Build history of the part. All positions in model axes, mm. A direction names the side the tool comes from. Round coordinates to 2 decimals unless told otherwise and drop trailing zeros. Write each loop counter-clockwise with the first axis right and the second up, starting at its lowest first coordinate (ties: lowest second). Pieces come first, ordered by that corner, then holes. Notation, with made-up numbers: (6, 0) -> (10, 0) arc R10 cw to (10, 12) -> close; hole circle Ø2 at (-23, -12.5). An arc over 180 degrees is marked (long way). One line per question, with ' | ' between items.
from build123d import *

# Parameters (mm, degrees)
SKETCH1_W               = 75
SKETCH1_H               = 30
BOSS_EXTRUDE1_DEPTH     = 3
SKETCH2_W               = 3
SKETCH2_H               = 30
BOSS_EXTRUDE2_DEPTH     = 7
SKETCH4_R               = 1.5
CUT_EXTRUDE1_DEPTH      = 3
MIRROR1_COPY_1_SKETCH_R = 1.5
MIRROR1_COPY_1_DEPTH    = 3
SKETCH5_W               = 16
SKETCH5_H               = 7
BOSS_EXTRUDE3_DEPTH     = 8
CHAMFER1_SIZE           = 5
CHAMFER1_SIZE2          = 7
CHAMFER2_SIZE           = 5
CHAMFER3_SIZE           = 2
SKETCH6_R               = 1.5
CUT_EXTRUDE2_DEPTH      = 8
CUT_EXTRUDE3_START      = -5
CUT_EXTRUDE3_DEPTH      = 42.149507332


with BuildPart() as part:
    # Sketch1 → Boss-Extrude1 (new body)
    with BuildSketch(Plane.XY):
        Rectangle(SKETCH1_W, SKETCH1_H)
    extrude(amount=BOSS_EXTRUDE1_DEPTH)

    # Sketch2 → Boss-Extrude2 (add)
    with BuildSketch(Plane(origin=(0, 0, 0), x_dir=(-1, 0, 0), z_dir=(0, 0, -1))):
        with Locations((-36, 0)):
            Rectangle(SKETCH2_W, SKETCH2_H)
    boss_extrude2 = extrude(amount=BOSS_EXTRUDE2_DEPTH)

    # Sketch4 → Cut-Extrude1 (cut)
    with BuildSketch(Plane.ZY.offset(-34.5)):
        with Locations((-4, 10)):
            Circle(SKETCH4_R)
    cut_extrude1 = extrude(amount=-CUT_EXTRUDE1_DEPTH, mode=Mode.SUBTRACT)

    # Mirror2: Cut-Extrude1 across plane
    add(cut_extrude1.mirror(Plane.ZX), mode=Mode.SUBTRACT)

    # Mirror1: Boss-Extrude2, Cut-Extrude1 across plane
    add(boss_extrude2.mirror(Plane(origin=(0, 0, 0), x_dir=(0, 0, 1), z_dir=(1, 0, 0))))
    add(cut_extrude1.mirror(Plane(origin=(0, 0, 0), x_dir=(0, 0, 1), z_dir=(1, 0, 0))), mode=Mode.SUBTRACT)

    # Mirror1 copy 1 sketch → Mirror1 copy 1 (cut)
    with BuildSketch(Plane(origin=(-34.5, 0, 0), x_dir=(0, 0, 1), z_dir=(1, 0, 0))):
        with Locations((-4, 10)):
            Circle(MIRROR1_COPY_1_SKETCH_R)
    extrude(amount=-MIRROR1_COPY_1_DEPTH, mode=Mode.SUBTRACT)

    # Sketch5 → Boss-Extrude3 (add)
    with BuildSketch(Plane.XZ.offset(15)):
        with Locations((0, -3.5)):
            Rectangle(SKETCH5_W, SKETCH5_H)
    extrude(amount=-BOSS_EXTRUDE3_DEPTH)

    # Chamfer1
    chamfer1_edges = [part.edges().sort_by_distance(p)[0] for p in [
        (0, -15, -7),
    ]]
    chamfer1_side = [part.faces().sort_by_distance(p)[0] for p in [
        (0, -11, -7),
    ]]
    chamfer(chamfer1_edges, length=CHAMFER1_SIZE, length2=CHAMFER1_SIZE2, reference=chamfer1_side[0])

    # Chamfer2
    chamfer2_edges = [part.edges().sort_by_distance(p)[0] for p in [
        (0, -7, 0),
    ]]
    chamfer(chamfer2_edges, length=CHAMFER2_SIZE)

    # Chamfer3
    chamfer3_edges = [part.edges().sort_by_distance(p)[0] for p in [
        (0, -7, -7),
    ]]
    chamfer(chamfer3_edges, length=CHAMFER3_SIZE - 0.0001)  # a hair under: the kernel refuses the full size

    # Sketch6 → Cut-Extrude2 (cut)
    with BuildSketch(Plane(origin=(0, -9.932432432, -7.094594595), x_dir=(1, 0, 0), z_dir=(0, -0.8137334712067358, -0.5812381937190955))):
        with Locations(Location((-4, 4.718572906, 0), (0, 0, 270))):
            Circle(SKETCH6_R)
        with Locations(Location((4, 4.718572906, 0), (0, 0, 270))):
            Circle(SKETCH6_R)
    extrude(amount=-CUT_EXTRUDE2_DEPTH, mode=Mode.SUBTRACT)

    # Sketch7 → Cut-Extrude3 (cut, through all)
    with BuildSketch(Plane(origin=(0, -9.932432432, -7.094594595), x_dir=(1, 0, 0), z_dir=(0, -0.8137334712067358, -0.5812381937190955)).offset(CUT_EXTRUDE3_START)):
        Polygon((-0.824573519, 4.718572906), (-2.41228676, 7.468572906), (-5.58771324, 7.468572906), (-7.175426481, 4.718572906), (-5.58771324, 1.968572906), (-2.41228676, 1.968572906), align=None)
        Polygon((7.175426481, 4.718572906), (5.58771324, 7.468572906), (2.41228676, 7.468572906), (0.824573519, 4.718572906), (2.41228676, 1.968572906), (5.58771324, 1.968572906), align=None)
    extrude(amount=-CUT_EXTRUDE3_DEPTH, mode=Mode.SUBTRACT)


solid = part.part
(1) Wall check: line 1 (Y direction, x = -35.85, z = -4); line 2 (X direction, y = -9.5, z = -5.5); line 3 (X direction, y = -7.25, z = -1.5). Give the ranges that are in metal, low to high. Write a range as from..to.
Calculated:
line 1: -15..-11.5, -8.5..8.5, 11.5..15 | line 2: -37.5..-34.5, -8..8, 34.5..37.5 | line 3: -37.5..-34.5, -8..-6.18, -1.82..1.82, 6.18..8, 34.5..37.5
(2) Slice it at B-B (y = 13). Write the cut outline in (x, z), then the cut area to 3 significant figures.
Calculated:
outline: (-37.5, -7) -> (-34.5, -7) -> (-34.5, 0) -> (34.5, 0) -> (34.5, -7) -> (37.5, -7) -> (37.5, 3) -> (-37.5, 3) -> close | area: 267 mm2
(3) Mould opens along X. For faces 1 (the cylindrical face through (-35.979, 9.425, -2.614)), 2 (the flat face through (-37.5, 0, -2)), 3 (the flat face through (8, -9, -3)) say: pulls with the +X half, pulls with the -X half, needs draft (parallel to the pull), parting line crosses it, or undercut.
Calculated:
face 1: needs draft | face 2: pulls with the -X half | face 3: undercut
(4) 3-axis set-ups, long thin cutter, end or side, ignore diameter. For faces 4 (the flat face through (-8, -9, -3)), 5 (the flat face through (-6.39, -4.83, 0.68)), 6 (the flat face through (0, -5, -3)): which of +Z, -Z, +X, -X, +Y, -Y reach the whole face in a straight line?
Calculated:
face 4: -Z, +Y, -Y | face 5: none | face 6: -Z, +Y
(5) Slice it at C-C (x = 9). Write the cut outline in (y, z).
Calculated:
outline: (-15, 0) -> (15, 0) -> (15, 3) -> (-15, 3) -> close
(6) Drop flat-ended pins along their axis: pin 1 (3.5 mm diameter, centred on y = -10, z = -4, fed in from +X); pin 2 (4 mm diameter, centred on x = 9.5, y = -6, fed in from -Z); pin 3 (3 mm diameter, centred on x = -2.5, y = 0, fed in from -Z). Give the stop position or say it passes through.
Calculated:
pin 1: x = 37.5 | pin 2: z = -5.32 | pin 3: z = 0
(7) Slice it at A-A (y = 10). Write the cut outline in (x, z).
Calculated:
outline: (-37.5, -7) -> (-34.5, -7) -> (-34.5, -5.5) -> (-37.5, -5.5) -> close; (-37.5, -2.5) -> (-34.5, -2.5) -> (-34.5, 0) -> (34.5, 0) -> (34.5, -2.5) -> (37.5, -2.5) -> (37.5, 3) -> (-37.5, 3) -> close; (34.5, -7) -> (37.5, -7) -> (37.5, -5.5) -> (34.5, -5.5) -> close
